```python
from build123d import *

# Parameters (mm, degrees)
PAD004_DEPTH = 1.2
SKETCH006_W  = 7.5
SKETCH006_H  = 8
PAD005_DEPTH = 5.6
SKETCH007_W  = 5.6
SKETCH007_H  = 7.6
PAD006_DEPTH = 2.9


with BuildPart() as part:
    # Sketch005 → Pad004 (new body)
    with BuildSketch(Plane.XY):
        Polygon((7, 11.75), (14.15, 11.75), (14.15, -11.75), (-14.15, -11.75), (-14.15, 14.85), (7, 14.85), align=None)
    extrude(amount=PAD004_DEPTH)

    # Sketch006 (on Face7 of Pad004) → Pad005 (join)
    with BuildSketch(Plane(origin=(0, 0, 0), x_dir=(1, 0, 0), z_dir=(0, 0, -1))):
        with Locations((10.4, -5)):
            Rectangle(SKETCH006_W, SKETCH006_H)
    extrude(amount=PAD005_DEPTH)

    # Sketch007 (on Face4 of Pad005) → Pad006 (join)
    with BuildSketch(Plane(origin=(0, 0, 0), x_dir=(1, 0, 0), z_dir=(0, 0, -1))):
        with Locations((11.35, 5.45)):
            Rectangle(SKETCH007_W, SKETCH007_H)
    extrude(amount=PAD006_DEPTH)


solid = part.part
```
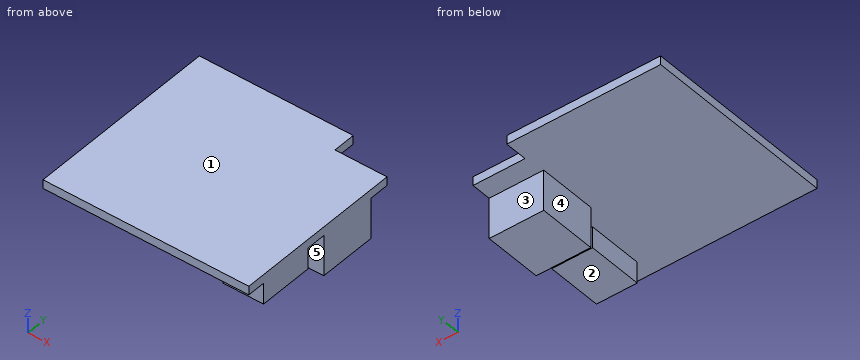
Verification items for the finished model (mm, model axes). Face numbers are marked on the shaded views. A direction names the side the tool comes from. Round coordinates to 2 decimals unless told otherwise and drop trailing zeros. Order: outer loops, then holes, each group sorted by start corner. A loop starts at its lowest first (then second) coordinate and runs counter-clockwise, first axis right, second up.
1) Tool access check on the marked faces 1 and 2. Record the directions out of +Z, -Z, +X, -X, +Y, -Y that give a thin tool (end or side, any length) a straight path to the whole face; none if there is none.
Geometry says:
face 1: +Z, +X, -X, +Y, -Y
face 2: -Z, +X, -X, -Y
2) Cross-section at D-D, the plane z = -4. Record the cut outline in (x, y).
Geometry says:
outline: (6.65, 1) - (14.15, 1) - (14.15, 9) - (6.65, 9) - close
3) Cross-section at C-C, the plane y = -5.5. Record the cut outline in (x, z).
Geometry says:
outline: (-14.15, 0) - (8.55, 0) - (8.55, -2.9) - (14.15, -2.9) - (14.15, 1.2) - (-14.15, 1.2) - close
4) Depth check by flat-ended pin: pin 1 (2 mm diameter, centred on y = 8, z = -2.5, fed in from -X); pin 2 (1.3 mm diameter, centred on y = 12.5, z = 0.5, fed in from +X); pin 3 (3 mm diameter, centred on x = 12, y = -6, fed in from -Z). Enter the tip coordinate at first touch or a pass-through.
Geometry says:
pin 1: stops at x = 6.65
pin 2: stops at x = 7
pin 3: stops at z = -2.9
5) Draft check along Y on the marked faces 3, 4 and 5. Enter one of: +Y half, -Y half, draft (parallel to the pull), parting line (faces both ways), or undercut.
Geometry says:
face 3: +Y half
face 4: draft
face 5: undercut
6) Material ranges on line 1 (Z direction, x = -9.25, y = -3.5); line 2 (Y direction, x = 10.5, z = -1); line 3 (X direction, y = 7, z = -4.5), recorded low to high.
Geometry says:
line 1: z = 0 to 1.2
line 2: y = -9.25 to -1.65, 1 to 9
line 3: x = 6.65 to 14.15
7) Cross-section at B-B, the plane x = 7.5. Record the cut outline in (y, z), plus the area to 3 significant figures.
Geometry says:
outline: (-11.75, 0) - (1, 0) - (1, -5.6) - (9, -5.6) - (9, 0) - (11.75, 0) - (11.75, 1.2) - (-11.75, 1.2) - close
area: 73.0 mm2
8) Cross-section at A-A, the plane z = -2. Record the cut outline in (x, y), plus the area to 3 significant figures.
Geometry says:
outline: (6.65, 1) - (14.15, 1) - (14.15, 9) - (6.65, 9) - close; (8.55, -9.25) - (14.15, -9.25) - (14.15, -1.65) - (8.55, -1.65) - close
area: 103 mm2
